For this review, take the finished solid that the model builds, in its own axes (mm). A direction names the side the tool comes from. Coordinates: 2 decimals unless noted, no trailing zeros. Loops run counter-clockwise (first coordinate to the right, second up) from the corner with the lowest first, then second, coordinate; pieces in that order, holes last. Notation, with made-up numbers: M 50,-24.75 L 71,-24.75 A32 cw 71,5.25 Z; hole C -1.5,-20.5 d7. An arc over 180 degrees is marked long. Answer as a JSON object with one key per item and string values. Group by question number.
Item 1: Wall thickness on L1, parallel to Y at x = 5, z = 4.25; L2, parallel to X at y = 6.75, z = 14; L3, parallel to Z at x = 46.5, y = 4: over which ranges is each line inside the solid? List them lowest first. Write a range as from..to.
Item 2: Add section B-B (x = 45). State the section outline as (y, z) points, then the cut area to 3 significant figures.
Item 3: Add section D-D (z = 12). State the section outline as (x, y) points, then the cut area to 3 significant figures.
Item 4: Tool access review of faces 1 (the face through (25, 10, 6)), 2 (the face through (15, 5, 14)), 3 (the face through (35, 5, 14)): name each direction out of +Z, -Z, +X, -X, +Y, -Y from which nothing blocks a thin tool from reaching the whole face with its end or side.
Item 5: Add section C-C (y = 5.5). State the section outline as (x, z) points.
Item 6: Insertion check: pin 1 (4 mm diameter, centred on y = 5, z = 17, fed in from +X); pin 2 (5 mm diameter, centred on y = 4.5, z = 13.5, fed in from -X); pin 3 (4 mm diameter, centred on x = 35, y = 9, fed in from +Z). Each pin has a flat end and moves straight along its axis. Give the tip position at first contact, or say it passes through.
Item 7: Mouldability with a two-part tool opening along Y and no side actions: class faces 4 (the face through (6.386, 4.425, 3.549)), 5 (the face through (25, 1, 20)), 6 (the face through (7, 5, 7)) as +Y half, -Y half, draft (parallel to the pull), parting line (faces both ways), or undercut.
from build123d import *

# Parameters (mm, degrees)
F0_W      = 50
F0_H      = 10
F1_DEPTH  = 7
F2_W      = 20
F2_H      = 10
F4_DEPTH  = 15
F5_R      = 4.99999
F3_R      = 1.5
F6_DEPTH  = 25
F7_R      = 1.5
F8_DEPTH  = 50
F10_W     = 10
F10_H     = 10
F11_DEPTH = 25


# Not quite as in the source:
# - a fillet or chamfer is up to 0.001 mm smaller than in the source, because OpenCascade refuses the exact size


with BuildPart() as f1:
    # F0 (on Top) → F1 (new body)
    with BuildSketch(Plane.XY):
        with Locations((25, 5)):
            Rectangle(F0_W, F0_H)
    extrude(amount=F1_DEPTH)

    # F2 (on face) → F4 (join)
    with BuildSketch(Plane.XY.offset(7)):
        with Locations((25, 5)):
            Rectangle(F2_W, F2_H)
    extrude(amount=F4_DEPTH)

    # F5 (radius 5 in the source; OpenCascade refuses exactly that, so slightly less here)
    f5_edges = [f1.edges().sort_by_distance(p)[0] for p in [
        (25, 10, 22),
        (25, 0, 22),
    ]]
    fillet(f5_edges, radius=F5_R)

    # F3 (on face) → F6 (cut)
    with BuildSketch(Plane.XY.offset(7)):
        with Locations((45, 5)):
            Circle(F3_R)
        with Locations((5, 5)):
            Circle(F3_R)
    extrude(amount=-F6_DEPTH, mode=Mode.SUBTRACT)

    # F7 (on face) → F8 (cut)
    with BuildSketch(Plane.YZ.offset(35)):
        with Locations((5, 17)):
            Circle(F7_R)
    extrude(amount=-F8_DEPTH, mode=Mode.SUBTRACT)


with BuildPart() as f9_1:
    # F9: copy of F1
    add(f1.part.moved(Location((0, 0, 40))))

    # F10 (on face) → F11 (cut)
    with BuildSketch(Plane.XY.offset(47)):
        with Locations((25, 5)):
            Rectangle(F10_W, F10_H)
    extrude(amount=F11_DEPTH, mode=Mode.SUBTRACT)


solid = f1.part
From the geometry:
{
 "1": {"L1": "y = 0..3.5, 6.5..10", "L2": "x = 15..35", "L3": "z = 0..7"},
 "2": {"outline": "M 0,0 L 3.5,0 L 3.5,7 L 0,7 Z; M 6.5,0 L 10,0 L 10,7 L 6.5,7 Z", "area": "49.0 mm²"},
 "3": {"outline": "M 15,0 L 35,0 L 35,10 L 15,10 Z", "area": "200 mm²"},
 "4": {"face 1": "+Z, -Z, +X, -X, +Y", "face 2": "+Z, -X, +Y, -Y", "face 3": "+Z, +X, +Y, -Y"},
 "5": {"outline": "M 0,0 L 3.59,0 L 3.59,7 L 0,7 Z; M 6.41,0 L 43.59,0 L 43.59,7 L 35,7 L 35,15.59 L 15,15.59 L 15,7 L 6.41,7 Z; M 15,18.41 L 35,18.41 L 35,21.97 L 15,21.97 Z; M 46.41,0 L 50,0 L 50,7 L 46.41,7 Z"},
 "6": {"pin 1": "stops at x = 35", "pin 2": "stops at x = 15", "pin 3": "stops at z = 21.58"},
 "7": {"face 4": "undercut", "face 5": "-Y half", "face 6": "draft"}
}
